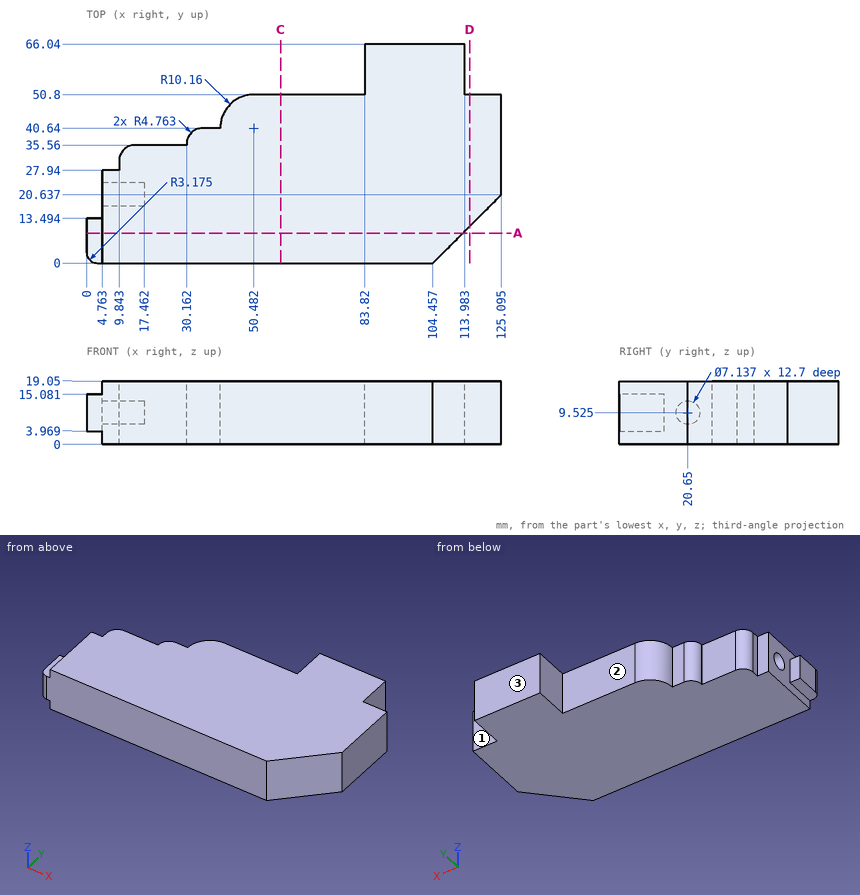
The figure shows three views and two pictorial views of one solid part (mm, origin at its lowest corner). Answer the questions. A direction names the side the tool comes from. Give positions to 0.01 mm unless a question says otherwise; leave off trailing zeros. Write each loop counter-clockwise with the first axis right and the second up, starting at its lowest first coordinate (ties: lowest second). Pieces come first, ordered by that corner, then holes. Notation, with made-up numbers: M -2,68 L 45,68 A18 ccw 45,80 Z; hole C -27,89 d8. An arc over 180 degrees is marked long. One line per item, written item: value. Start each with the question number.
(1) A tool of negligible diameter and unlimited length cuts with its end or side. For the marked faces 1, 2 and 3, from which of +Z, -Z, +X, -X, +Y, -Y can it reach the whole face along a straight path? Write none if from no direction.
(2) Find section A-A (y = 9). Determine the outline of the cut face in (x, z), plus the area to 3 significant figures.
(3) Flat-ended cylindrical pins translate along their axes: pin 1 Ø4 at (x, y) = (1.5, 9) entering from -Z; pin 2 Ø4.5 at (y, z) = (20.65, 9.52) entering from -X; pin 3 Ø1.5 at (x, z) = (6, 14) entering from +Y. Find the tip coordinate at first contact, or state that the pin passes through.
(4) Find the intervals of material crossed by line 1 (Y direction, x = 20, z = 6.5); line 2 (Y direction, x = 40, z = 9.5); line 3 (X direction, y = 59, z = 8), in increasing order.
(5) Find section C-C (x = 58.5). Determine the outline of the cut face in (y, z).
(6) Find section D-D (x = 115.5). Determine the outline of the cut face in (y, z).
Results below:
1. face 1: +Z, -Z, +X, +Y
1. face 2: +Z, -Z, -X, +Y
1. face 3: +Z, -Z, +X, -X, +Y
2. outline: M 0,3.97 L 4.76,3.97 L 4.76,0 L 113.46,0 L 113.46,19.05 L 4.76,19.05 L 4.76,15.08 L 0,15.08 Z
2. area: 2,120 mm^2
3. pin 1: stops at z = 3.97
3. pin 2: stops at x = 17.46
3. pin 3: stops at y = 27.94
4. line 1: y = 0 to 35.56
4. line 2: y = 0 to 40.64
4. line 3: x = 83.82 to 113.98
5. outline: M 0,0 L 50.8,0 L 50.8,19.05 L 0,19.05 Z
6. outline: M 11.04,0 L 50.8,0 L 50.8,19.05 L 11.04,19.05 Z
